Autodesk Inventor part; units mm, degrees
ref_plane "YZ Plane" through (0, 0, 0) normal (1, 0, 0) x (0, 1, 0)
ref_plane "XZ Plane" through (0, 0, 0) normal (0, 1, 0) x (-1, 0, 0)
ref_plane "XY Plane" through (0, 0, 0) normal (0, 0, 1) x (1, 0, 0)
sketch "Sketch1" plane through (0, 0, 0) normal (0, 0, 1) x (1, 0, 0)
  line L0 (-77.7875, -41.275) -> (77.7875, -41.275)
  line L1 (77.7875, -41.275) -> (77.7875, 41.275)
  line L2 (77.7875, 41.275) -> (-77.7875, 41.275)
  line L3 (-77.7875, 41.275) -> (-77.7875, -41.275)
  line L4 (-77.7875, -41.275) -> (77.7875, 41.275) construction
  line L5 (77.7875, -41.275) -> (-77.7875, 41.275) construction
  point P0 (0, 0)
  dimension "d0" = 155.575
  dimension "d1" = 82.55
extrude "Extrusion1" add sketch "Sketch1" along normal blind 6.35
sketch "Sketch2" plane through (0, 0, 0) normal (0, 0, -1) x (-1, 0, 0)
  line L0 (-74.6125, -28.575) -> (74.6125, -28.575)
  line L1 (74.6125, -28.575) -> (74.6125, 28.575)
  line L2 (74.6125, 28.575) -> (-74.6125, 28.575)
  line L3 (-74.6125, 28.575) -> (-74.6125, -28.575)
  line L4 (-74.6125, -28.575) -> (74.6125, 28.575) construction
  line L5 (74.6125, -28.575) -> (-74.6125, 28.575) construction
  point P0 (0, 0)
  dimension "d4" = 149.225
  dimension "d5" = 57.15
hole "Hole1" at (74.6125, 28.575, 0) at (74.6125, -28.575, 0) at (-74.6125, 28.575, 0) at (-74.6125, -28.575, 0) direction (0, 0, 1) diameter 3.81 end through all counterbore diameter 7.1374 counterbore depth 3.5052
properties part number "front"
Geometry check sheet. Reference: the model listing, model coordinates, mm. A direction names the side the tool comes from. Give positions to 0.01 mm unless a question says otherwise; leave off trailing zeros. Order: outer loops, then holes, each group sorted by start corner. A loop starts at its lowest first (then second) coordinate and runs counter-clockwise, first axis right, second up. Notation, with made-up numbers: (53.25, 25) - (97.25, 25) arc R25 cw to (97.25, 54) - close; hole circle Ø10 at (-13, -29.75). An arc over 180 degrees is marked (long way). Write item = value, one per line. Start each with the question number.
1) Access from +Z, -Z, +X, -X, +Y, -Y to the whole of each face (thin tool, end or side, straight path). Record for faces 5 (the flat face through (75.9, -30.2, 3.505)), 6 (the flat face through (-1, 1, 6.35)).
2) Scan lines: L1, parallel to X at y = -27.5, z = 5; L2, parallel to X at y = -29, z = 5.25. Record each from-to range of solid material in increasing order.
3) Section check A-A (y = 28.5). Enter the section's corners in (x, z), then the cut area to 3 significant figures.
4) Gauge pin test, flat end, axial feed: pin 1 Ø2 at (x, y) = (-76, 29) entering from -Z. Record the tip position at first contact, or that the pin passes through.
5) Draft check along Y on faces 1 (the flat face through (1, 41.275, 3)), 2 (the flat face through (-76, 30.1, 3.505)), 3 (the cylindrical face through (-75.9, 27.17, 4.95)), 4 (the flat face through (-77.788, 1, 3)). Enter one of: released by +Y, released by -Y, zero draft, split by the parting line, or undercut.
Geometry check:
q1.face_5 = -Z
q1.face_6 = +Z, +X, -X, +Y, -Y
q2.L1 = -77.79 to -76.19, -73.04 to 73.04, 76.19 to 77.79
q2.L2 = -77.79 to -76.47, -72.76 to 72.76, 76.47 to 77.79
q3.outline = (-77.79, 3.51) - (-76.52, 3.51) - (-76.52, 6.35) - (-77.79, 6.35) - close; (-72.71, 3.51) - (-71.04, 3.51) - (-71.04, 0) - (71.04, 0) - (71.04, 3.51) - (72.71, 3.51) - (72.71, 6.35) - (-72.71, 6.35) - close; (76.52, 3.51) - (77.79, 3.51) - (77.79, 6.35) - (76.52, 6.35) - close
q3.area = 919 mm2
q4.pin_1 = 3.51
q5.face_1 = released by +Y
q5.face_2 = undercut
q5.face_3 = undercut
q5.face_4 = zero draft
